from build123d import *

# Parameters (mm, degrees)
F0_W     = 10.922
F0_H     = 25.7175
F1_DEPTH = 12.7
F2_W     = 6.604
F2_H     = 20.6375
F3_DEPTH = 25.4
F5_DEPTH = 32.18438
F6_R     = 1.27
F7_DEPTH = 25.4
F8_SIZE  = 1.27


with BuildPart() as f1:
    # F0 (on Top) → F1 (new body)
    with BuildSketch(Plane.XY):
        Rectangle(F0_W, F0_H)
    extrude(amount=F1_DEPTH)

    # F2 (on face) → F3 (cut)
    with BuildSketch(Plane.XY.offset(12.7)):
        Rectangle(F2_W, F2_H)
    extrude(amount=-F3_DEPTH, mode=Mode.SUBTRACT)

    # F4 (on face) → F5 (cut)
    with BuildSketch(Plane(origin=(0, 12.85875, 0), x_dir=(-1, 0, 0), z_dir=(0, 1, 0))):
        Polygon((0, 12.7), (-3.302, 12.7), (-3.302, 3.175), (3.302, 3.175), (3.302, 12.7), align=None)
    extrude(amount=-F5_DEPTH, mode=Mode.SUBTRACT)

    # F6 (on face) → F7 (cut)
    with BuildSketch(Plane.YZ.offset(5.461)):
        with Locations((-4.7625, 3.172593)):
            Circle(F6_R)
        with Locations((4.7625, 3.172593)):
            Circle(F6_R)
    extrude(amount=-F7_DEPTH, mode=Mode.SUBTRACT)

    # F8
    f8_edges = [f1.edges().sort_by_distance(p)[0] for p in [
        (-5.461, 0, 12.7),
        (5.461, 0, 12.7),
        (4.3815, 12.85875, 12.7),
        (-4.3815, 12.85875, 12.7),
        (4.3815, -12.85875, 12.7),
        (-4.3815, -12.85875, 12.7),
    ]]
    chamfer(f8_edges, length=F8_SIZE)


solid = f1.part
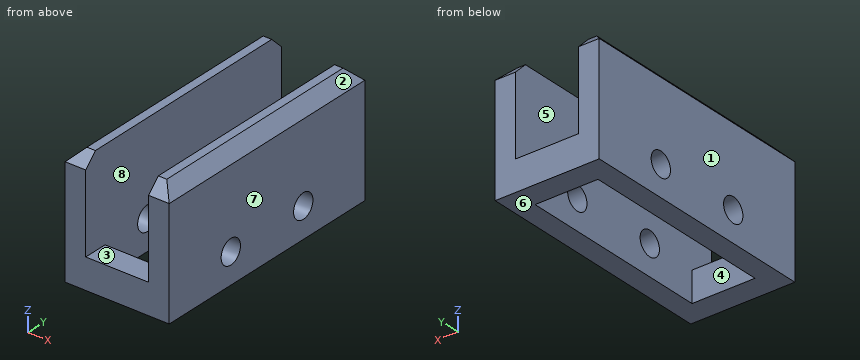
For this review, take the finished solid that the model builds, in its own axes (mm). Face numbers are marked on the shaded views. A direction names the side the tool comes from. Round coordinates to 2 decimals unless told otherwise and drop trailing zeros. Order: outer loops, then holes, each group sorted by start corner. A loop starts at its lowest first (then second) coordinate and runs counter-clockwise, first axis right, second up. Notation, with made-up numbers: (38, 52.5) -> (50, 52.5) arc R10 cw to (50, 58.5) -> close; hole circle Ø3 at (65.5, 78). An arc over 180 degrees is marked (long way). Write item = value, one per line. Start each with the question number.
1) Take a section at C-C on y = -0.25. State the section outline as (x, z) points.
2) The part is to be moulded in two halves that separate along X. For the marked faces 6, 7 and 8, say which applies: +X half, -X half, draft (parallel to the pull), parting line (faces both ways), or undercut.
3) Tool access review of the marked faces 1, 2, 3, 4 and 5: name each direction out of +Z, -Z, +X, -X, +Y, -Y from which nothing blocks a thin tool from reaching the whole face with its end or side.
4) Take a section at D-D on z = 4. State the section outline as (x, y) points, plus the area to 3 significant figures.
5) Take a section at A-A on z = 9.75. State the section outline as (x, y) points.
6) Take a section at B-B on x = 1.75. State the section outline as (y, z) points (3 decimals), plus the area to 3 significant figures.
7) To check wall thickness, follow line 1 (Y direction, x = -2, z = 2.25); line 2 (X direction, y = 5.75, z = 5.25); line 3 (Y direction, x = 4.75, z = 3.25). State the ranges of each line that lie inside material, in increasing order. Write a range as from..to.
8) Insertion check: pin 1 (3.5 mm diameter, centred on y = 4.76, z = 3.17, fed in from -X); pin 2 (1.3 mm diameter, centred on x = 0.5, y = -12, fed in from +Z) (3 decimals). Each pin has a flat end and moves straight along its axis. Give the tip position at first contact, or say it passes through.
Verdict:
q1.outline = (-5.46, 0) -> (-3.3, 0) -> (-3.3, 12.7) -> (-4.19, 12.7) -> (-5.46, 11.43) -> close; (3.3, 0) -> (5.46, 0) -> (5.46, 11.43) -> (4.19, 12.7) -> (3.3, 12.7) -> close
q2.face_6 = draft
q2.face_7 = +X half
q2.face_8 = undercut
q3.face_1 = +Z, -Z, -X, +Y, -Y
q3.face_2 = +Z, +X, +Y, -Y
q3.face_3 = +Z, +Y, -Y
q3.face_4 = +Z, -Z
q3.face_5 = +Z
q4.outline = (-5.46, -12.86) -> (-3.3, -12.86) -> (-3.3, -5.73) -> (-5.46, -5.73) -> close; (-5.46, -3.8) -> (-3.3, -3.8) -> (-3.3, 3.8) -> (-5.46, 3.8) -> close; (-5.46, 5.73) -> (-3.3, 5.73) -> (-3.3, 12.86) -> (-5.46, 12.86) -> close; (3.3, -12.86) -> (5.46, -12.86) -> (5.46, -5.73) -> (3.3, -5.73) -> close; (3.3, -3.8) -> (5.46, -3.8) -> (5.46, 3.8) -> (3.3, 3.8) -> close; (3.3, 5.73) -> (5.46, 5.73) -> (5.46, 12.86) -> (3.3, 12.86) -> close
q4.area = 94.4 mm2
q5.outline = (-5.46, -12.86) -> (-3.3, -12.86) -> (-3.3, 12.86) -> (-5.46, 12.86) -> close; (3.3, -12.86) -> (5.46, -12.86) -> (5.46, 12.86) -> (3.3, 12.86) -> close
q6.outline = (-12.859, 0) -> (-10.319, 0) -> (-10.319, 3.175) -> (-12.859, 3.175) -> close; (10.319, 0) -> (12.859, 0) -> (12.859, 3.175) -> (10.319, 3.175) -> close
q6.area = 16.1 mm2
q7.line_1 = -12.86..-10.32, 10.32..12.86
q7.line_2 = -5.46..-3.3, 3.3..5.46
q7.line_3 = -12.86..-6.03, -3.49..3.49, 6.03..12.86
q8.pin_1 = -5.46
q8.pin_2 = 3.175
